The model under review builds one solid part; all positions refer to its coordinate system, in mm. Face numbers are marked on the shaded views. A direction names the side the tool comes from. Coordinates: 2 decimals unless noted, no trailing zeros. Loops run counter-clockwise (first coordinate to the right, second up) from the corner with the lowest first, then second, coordinate; pieces in that order, holes last. Notation, with made-up numbers: (64.25, 3.5) - (109.25, 3.5) arc R22 cw to (109.25, 42.5) - close; hole circle Ø7 at (18.5, -24). An arc over 180 degrees is marked (long way). Answer in a Markdown table with one row per item. Add a question column.
(1) We need section A-A on y = 99.5. Write out the cut boundary in (x, z) (3 decimals).
(2) Mouldability with a two-part tool opening along Z and no side actions: class the marked faces 4, 5 and 6 as +Z half, -Z half, draft (parallel to the pull), parting line (faces both ways), or undercut.
(3) We need section D-D on z = 81. Write out the cut boundary in (x, y), plus the area to 3 significant figures.
(4) We need section C-C on x = 33.02. Write out the cut boundary in (y, z) (3 decimals).
(5) For P1, Ø3, axis at x = 34, z = 110.5, coming from the -Y side; P2, Ø1, axis at x = 47, z = 37, coming from the +Y side; P3, Ø7, axis at y = 57.823, z = 63.5, coming from the -X side, all flat-tipped, find the tip position at first contact; note any pin that passes through.
(6) We need section B-B on z = 63.5. Write out the cut boundary in (x, y) (3 decimals), plus the area to 3 significant figures.
(7) Machinability: for the marked faces 1, 2 and 3, which of the approach directions +Z, -Z, +X, -X, +Y, -Y give a long, thin tool a straight path to every point of the face, cutting with its end or side? Answer none if there is none.
(8) For line 1 along X through (y, z) = (85, 7) (3 decimals); line 2 along Y through (x, z) = (10, 9); line 3 along X through (y, z) = (64.5, 117), list the stretches that pass through material, from the lowest coordinate up.
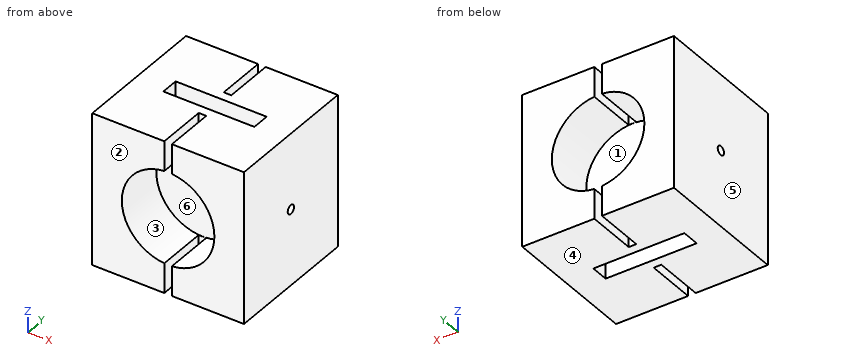
Autodesk Fusion 360 part; units mm, degrees
sketch "Sketch1" plane through (0, 0, 0) normal (0, 0, 1) x (1, 0, 0)
  line L0 (-30.48, 114.973) -> (96.52, 114.973)
  line L1 (96.52, 114.973) -> (96.52, 0.673)
  line L2 (96.52, 0.673) -> (-30.48, 0.673)
  line L3 (-30.48, 0.673) -> (-30.48, 114.973)
  line L4 (-5.08, 65.323) -> (71.12, 65.323)
  line L5 (71.12, 65.323) -> (71.12, 50.323)
  line L6 (71.12, 50.323) -> (-5.08, 50.323)
  line L7 (-5.08, 50.323) -> (-5.08, 65.323)
  line L8 (29.845, 114.973) -> (36.195, 114.973)
  line L9 (36.195, 114.973) -> (36.195, 73.063)
  line L10 (36.195, 73.063) -> (29.845, 73.063)
  line L11 (29.845, 73.063) -> (29.845, 114.973)
  line L12 (29.845, 0.673) -> (36.195, 0.673)
  line L13 (36.195, 0.673) -> (36.195, 42.583)
  line L14 (36.195, 42.583) -> (29.845, 42.583)
  line L15 (29.845, 42.583) -> (29.845, 0.673)
  dimension "d1" = 114.3
  dimension "d2" = 127
  dimension "d3" = 15
  dimension "d4" = 76.2
  dimension "d5" = 25.4
  dimension "d8" = 49.65
  dimension "d9" = 6.35
  dimension "d10" = 60.325
  dimension "d11" = 41.91
  dimension "d12" = 41.91
  dimension "d13" = 60.325
  dimension "d14" = 6.35
extrude "Extrude1" add sketch "Sketch1" along normal blind 127 contours L0 L1 L2 L3 L9 L10 L11 L13 L14 L15
sketch "Sketch2" plane through (0, 0.673, 0) normal (0, -1, 0) x (1, 0, 0)
  line L0 (-30.48, 0) -> (29.845, 0)
  line L1 (29.845, 0) -> (29.845, 127)
  line L2 (29.845, 127) -> (-30.48, 127)
  line L3 (-30.48, 127) -> (-30.48, 0)
  circle A0 centre (33.02, 63.5) radius 38.735
  dimension "d17" = 77.47
  dimension "d18" = 63.5
  dimension "d19" = 63.5
extrude "Extrude2" cut sketch "Sketch2" against normal blind 42.037 contours L1 A0 | L1 A0
sketch "Sketch3" plane through (0, 114.973, 0) normal (0, 1, 0) x (-1, 0, 0)
  line L0 (-29.845, 0) -> (30.48, 0)
  line L1 (30.48, 0) -> (30.48, 127)
  line L2 (30.48, 127) -> (-29.845, 127)
  line L3 (-29.845, 127) -> (-29.845, 0)
  circle A0 centre (-33.02, 63.5) radius 38.735
  dimension "d22" = 77.47
  dimension "d23" = 63.5
  dimension "d24" = 63.5
extrude "Extrude3" cut sketch "Sketch3" against normal blind 42.037 contours L3 A0 | L3 A0
sketch "Sketch4" plane through (96.52, 0, 0) normal (1, 0, 0) x (0, 1, 0)
  line L0 (0.673, 0) -> (114.973, 0)
  line L1 (114.973, 0) -> (114.973, 127)
  line L2 (114.973, 127) -> (0.673, 127)
  line L3 (0.673, 127) -> (0.673, 0)
  circle A0 centre (57.823, 63.5) radius 3.81
  dimension "d39" = 7.62
  dimension "d40" = 63.5
  dimension "d41" = 57.15
extrude "Extrude4" cut sketch "Sketch4" against normal blind 127 contours A0
Outcome:
| question | item | result |
|---|---|---|
| 1 | outline | (-30.48, 0) - (29.845, 0) - (29.845, 24.895) arc R38.735 cw to (29.845, 102.105) - (29.845, 127) - (-30.48, 127) - close; (36.195, 0) - (96.52, 0) - (96.52, 127) - (36.195, 127) - (36.195, 102.105) arc R38.735 cw to (36.195, 24.895) - close |
| 2 | face 4 | -Z half |
| 2 | face 5 | draft |
| 2 | face 6 | undercut |
| 3 | outline | (-30.48, 0.67) - (-1.54, 0.67) - (-1.54, 42.71) - (67.58, 42.71) - (67.58, 0.67) - (96.52, 0.67) - (96.52, 114.97) - (67.58, 114.97) - (67.58, 72.94) - (-1.54, 72.94) - (-1.54, 114.97) - (-30.48, 114.97) - close; hole (-5.08, 50.32) - (71.12, 50.32) - (71.12, 65.32) - (-5.08, 65.32) - close |
| 3 | area | 7,560 mm² |
| 4 | outline | (42.583, 0) - (50.323, 0) - (50.323, 127) - (42.583, 127) - (42.583, 102.235) - (42.71, 102.235) - (42.71, 24.765) - (42.583, 24.765) - close; (65.323, 0) - (73.063, 0) - (73.063, 24.765) - (72.936, 24.765) - (72.936, 102.235) - (73.063, 102.235) - (73.063, 127) - (65.323, 127) - close |
| 5 | P1 | y = 42.58 |
| 5 | P2 | y = 72.94 |
| 5 | P3 | through |
| 6 | outline | (-30.48, 0.673) - (-5.715, 0.673) - (-5.715, 42.71) - (71.755, 42.71) - (71.755, 0.673) - (96.52, 0.673) - (96.52, 54.013) - (71.12, 54.013) - (71.12, 50.323) - (-5.08, 50.323) - (-5.08, 54.013) - (-30.48, 54.013) - close; (-30.48, 61.633) - (-5.08, 61.633) - (-5.08, 65.323) - (71.12, 65.323) - (71.12, 61.633) - (96.52, 61.633) - (96.52, 114.973) - (71.755, 114.973) - (71.755, 72.936) - (-5.715, 72.936) - (-5.715, 114.973) - (-30.48, 114.973) - close |
| 6 | area | 6,470 mm² |
| 7 | face 1 | +Y |
| 7 | face 2 | +Z, -Z, +X, -X, -Y |
| 7 | face 3 | -Y |
| 8 | line 1 | -30.48 to 29.845, 36.195 to 96.52 |
| 8 | line 2 | 0.67 to 50.32, 65.32 to 114.97 |
| 8 | line 3 | -30.48 to -5.08, 71.12 to 96.52 |
